Geometry: see drawing. Coordinates: mm, zero at the bounding-box minimum. A direction names the side the tool comes from. Round coordinates to 2 decimals unless told otherwise and drop trailing zeros. Loops run counter-clockwise (first coordinate to the right, second up) from the corner with the lowest first, then second, coordinate; pieces in that order, holes last. Notation, with made-up numbers: (12.25, 89) - (44.25, 89) arc R30 ccw to (44.25, 119) - close; hole circle Ø6 at (-6, 43). An arc over 180 degrees is marked (long way). Return JSON: item names as keys, results as strings. Group by question number.
1. Material intervals for probe 1 along Z at (x, y) = (13.75, 4.5); probe 2 along X at (y, z) = (1, 19) (1 decimal), sorted ascending.
2. Draft query along Z for the marked faces 4, 5, 6 and 7. Return one class per face: +Z half, -Z half, draft (parallel to the pull), parting line (faces both ways), or undercut.
3. Section C-C on x = 12.7. Return loops of the section in (y, z) (1 decimal).
4. Section A-A on z = 12.7. Return loops of the section in (x, y) (1 decimal).
5. Set-up query: the marked faces 1, 2 and 3. Return all of +Z, -Z, +X, -X, +Y, -Y with unobstructed straight access to the full face (end or side cutting, diameter ignored); none if empty.
6. Section D-D on x = 8.5. Return loops of the section in (y, z) (1 decimal).
7. First-contact query: pin 1 Ø10 at (x, z) = (15, 14.5) entering from +Y (1 decimal). Flat tip, straight axial feed; report the tip coordinate or a pass-through.
8. Section B-B on y = 6.5. Return loops of the section in (x, z), and give its area (3 significant figures).
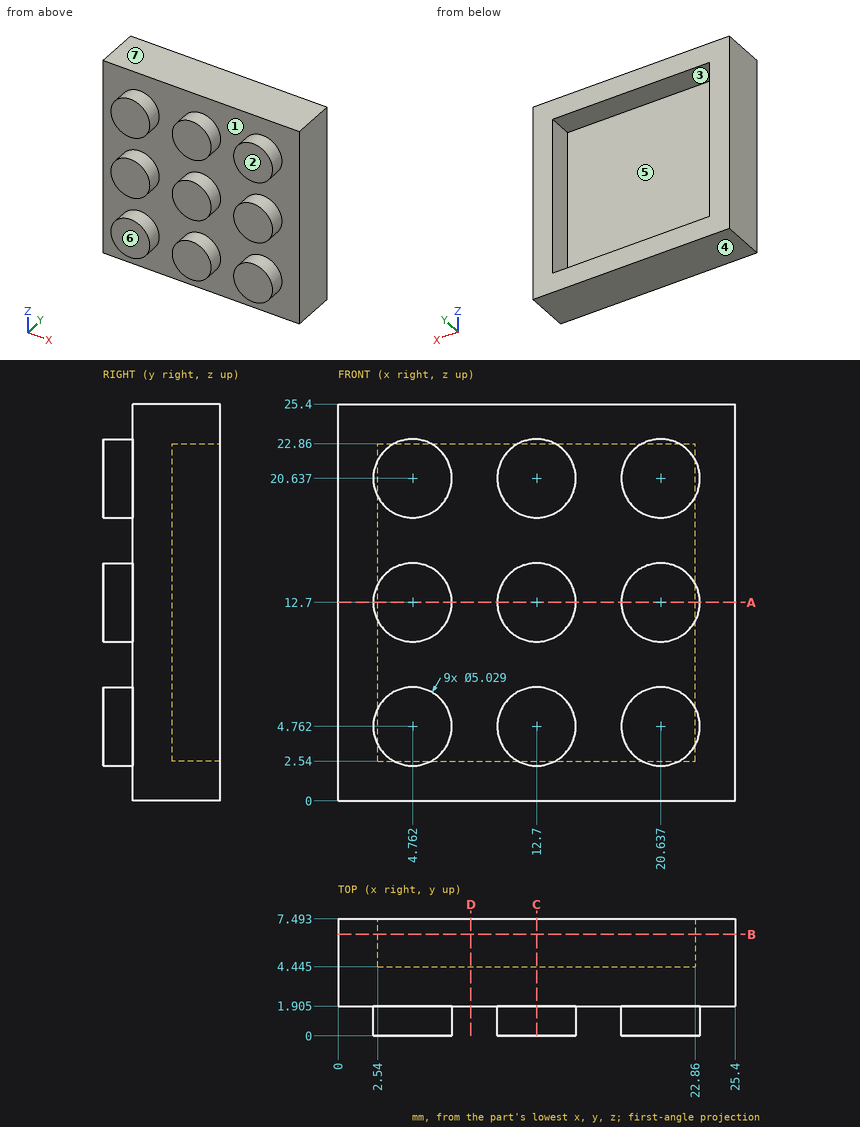
Taken from the geometry:
{
 "1": {"probe 1": "0 to 2.54, 22.86 to 25.4", "probe 2": "2.9 to 6.7, 10.8 to 14.6, 18.7 to 22.5"},
 "2": {"face 4": "-Z half", "face 5": "undercut", "face 6": "draft", "face 7": "+Z half"},
 "3": {"outline": "(0, 2.2) - (1.9, 2.2) - (1.9, 0) - (7.5, 0) - (7.5, 2.5) - (4.4, 2.5) - (4.4, 22.9) - (7.5, 22.9) - (7.5, 25.4) - (1.9, 25.4) - (1.9, 23.2) - (0, 23.2) - (0, 18.1) - (1.9, 18.1) - (1.9, 15.2) - (0, 15.2) - (0, 10.2) - (1.9, 10.2) - (1.9, 7.3) - (0, 7.3) - close"},
 "4": {"outline": "(0, 1.9) - (2.2, 1.9) - (2.2, 0) - (7.3, 0) - (7.3, 1.9) - (10.2, 1.9) - (10.2, 0) - (15.2, 0) - (15.2, 1.9) - (18.1, 1.9) - (18.1, 0) - (23.2, 0) - (23.2, 1.9) - (25.4, 1.9) - (25.4, 7.5) - (22.9, 7.5) - (22.9, 4.4) - (2.5, 4.4) - (2.5, 7.5) - (0, 7.5) - close"},
 "5": {"face 1": "-Y", "face 2": "+Z, -Z, +X, -X, -Y", "face 3": "+Y"},
 "6": {"outline": "(1.9, 0) - (7.5, 0) - (7.5, 2.5) - (4.4, 2.5) - (4.4, 22.9) - (7.5, 22.9) - (7.5, 25.4) - (1.9, 25.4) - close"},
 "7": {"pin 1": "y = 4.4"},
 "8": {"outline": "(0, 0) - (25.4, 0) - (25.4, 25.4) - (0, 25.4) - close; hole (2.54, 2.54) - (22.86, 2.54) - (22.86, 22.86) - (2.54, 22.86) - close", "area": "232 mm2"}
}
